Could you check a few things on this model? Use its own coordinates, in mm. Give positions to 0.01 mm unless a question says otherwise; leave off trailing zeros. Loops run counter-clockwise (first coordinate to the right, second up) from the corner with the lowest first, then second, coordinate; pieces in that order, holes last. Notation, with made-up numbers: (73, 45) -> (96, 45) arc R21 ccw to (96, 74) -> close; hole circle Ø7 at (70.25, -38.75). An arc over 180 degrees is marked (long way). Write item = value, one per line. Start each with the question number.
1) I want a section at D-D (x = -24). List the corners of the cut face in (y, z) for me.
2) I want a section at B-B (y = 25.5). List the corners of the cut face in (x, z) for me.
3) I'm going to push flat-ended pins straight in: pin 1 Ø18 at (x, y) = (0, 0) entering from +Z; pin 2 Ø3 at (y, z) = (28.5, 4.5) entering from -X. Where does each tip first touch, or does it pass through?
4) I want a section at A-A (x = 4). List the corners of the cut face in (y, z) for me.
5) I want a section at C-C (z = 5.5). List the corners of the cut face in (x, y) for me.
6) If we mould it in two halves opening along X, with no side actions, what happens to faces 1 (the face through (13.93, 40.2, 3.45)), 2 (the face through (-0.4, 11.4, 0)), 3 (the face through (-11.19, 0.49, 3.45))? For each: +X half, -X half, draft (parallel to the pull), parting line (faces both ways), or undercut.
7) I need wall thicknesses on probe 1 along Y at (x, z) = (-14, 5.75); probe 2 along Y at (x, z) = (0, 5.75); probe 3 along Y at (x, z) = (-2.5, 6). Which ranges of each line are inside material? Lowest first, please. Write a range as from..to.
from build123d import *

# Parameters (mm, degrees)
F0_R         = 11.2
F1_DEPTH     = 7
F2_T4_ANGLE  = 151.1667099625
F2_T10_ANGLE = 155.7575231718
F2_T16_ANGLE = 151.1667099625
F2_T22_ANGLE = 155.7575231718


# Not quite as in the source:
# - a fillet or chamfer that OpenCascade refuses, or shapes differently, is made with other operations: its cross-section is extruded or revolved along the edge and cut away or added


with BuildPart() as f1:
    # F0 (on Top) → F1 (new body)
    with BuildSketch(Plane.XY):
        with BuildLine():
            ThreePointArc((9.3591465956, -16.7270162039), (17.6571466732, 0.0595617509), (8.3139799998, 16.2876621091))
            Line((8.3139799998, 16.2876621091), (-9.3591465956, 16.7270162039))
            ThreePointArc((-9.3591465956, 16.7270162039), (-17.3223324531, -0.048962325), (-8.3139799998, -16.2876621091))
            Line((-8.3139799998, -16.2876621091), (9.3591465956, -16.7270162039))
        make_face()
        Circle(F0_R, mode=Mode.SUBTRACT)
        Polygon((8.3139799998, 16.2876621091), (27.5946892798, 32.5588136911), (-0.1261595724, 48.0615143736), (-27.5946892798, 33.4348380566), (-9.3591465956, 16.7270162039), align=None)
        with Locations((0, 31.6827967763)):
            Circle(F0_R, mode=Mode.SUBTRACT)
        Polygon((27.5946892798, -33.4348380566), (9.3591465956, -16.7270162039), (-8.3139799998, -16.2876621091), (-27.5946892798, -32.5588136911), (0.1261595724, -48.0615143736), align=None)
        with Locations((0, -31.6827967763)):
            Circle(F0_R, mode=Mode.SUBTRACT)
    extrude(amount=F1_DEPTH)

    # F2: fillet of radius 3 on 4 edges, made by hand


with BuildPart() as f2_tool2:
    # F2_s3 → F2_t4 (revolve)
    with BuildSketch(Plane(origin=(2.9031932082, 0.8450981198, 0), x_dir=(0, 0, 1), z_dir=(0.9601480198, 0.2794920035, 0))):
        with BuildLine():
            ThreePointArc((4, -20.0470026749), (6.1213203436, -19.1683230184), (7, -17.0470026749))
            Line((7, -17.0470026749), (7, -20.0470026749))
            Line((7, -20.0470026749), (4, -20.0470026749))
        make_face()
    revolve(axis=Axis((2.9763887281, 0.5936471566, 7), (0, 0, 1)), revolution_arc=F2_T4_ANGLE)

    split(bisect_by=Plane(origin=(4.0604237069, 4.4316985467, 0), x_dir=(0, 0, 1), z_dir=(-0.6755468125, -0.7373170987, 0)), keep=Keep.TOP)

    split(bisect_by=Plane(origin=(4.569745577, -5.414978498, 0), x_dir=(0, 0, 1), z_dir=(-0.6449416276, 0.7642318346, 0)), keep=Keep.TOP)


with BuildPart() as f1_1:
    add(f1.part)

    # F2_t1: cut F2_tool2
    add(f2_tool2.part, mode=Mode.SUBTRACT)


with BuildPart() as f2_tool8:
    # F2_s9 → F2_t10 (revolve)
    with BuildSketch(Plane(origin=(-2.2049800931, -0.547085883, 0), x_dir=(0, 0, 1), z_dir=(-0.9705717322, -0.2408121936, 0))):
        with BuildLine():
            ThreePointArc((4, -19.889257837), (6.1213203436, -19.0105781805), (7, -16.889257837))
            Line((7, -16.889257837), (7, -19.889257837))
            Line((7, -19.889257837), (4, -19.889257837))
        make_face()
    revolve(axis=Axis((-2.1995295918, -0.5690536346, 7), (0, 0, 1)), revolution_arc=F2_T10_ANGLE)

    split(bisect_by=Plane(origin=(-4.0604237069, -4.4316985467, 0), x_dir=(0, 0, 1), z_dir=(0.6755468125, 0.7373170987, 0)), keep=Keep.TOP)

    split(bisect_by=Plane(origin=(-4.569745577, 5.414978498, 0), x_dir=(0, 0, 1), z_dir=(0.6449416276, -0.7642318346, 0)), keep=Keep.TOP)


with BuildPart() as f1_2:
    add(f1_1.part)

    # F2_t7: cut F2_tool8
    add(f2_tool8.part, mode=Mode.SUBTRACT)


with BuildPart() as f2_tool14:
    # F2_s15 → F2_t16 (revolve)
    with BuildSketch(Plane(origin=(2.9031932082, 0.8450981198, 0), x_dir=(0, 0, 1), z_dir=(0.9601480198, 0.2794920035, 0))):
        with BuildLine():
            ThreePointArc((3, -20.0470026749), (0.8786796564, -19.1683230184), (0, -17.0470026749))
            Line((0, -17.0470026749), (0, -20.0470026749))
            Line((0, -20.0470026749), (3, -20.0470026749))
        make_face()
    revolve(axis=Axis((2.9763887281, 0.5936471566, 0), (0, 0, 1)), revolution_arc=F2_T16_ANGLE)

    split(bisect_by=Plane(origin=(4.0604237069, 4.4316985467, 0), x_dir=(0, 0, 1), z_dir=(-0.6755468125, -0.7373170987, 0)), keep=Keep.TOP)

    split(bisect_by=Plane(origin=(4.569745577, -5.414978498, 0), x_dir=(0, 0, 1), z_dir=(-0.6449416276, 0.7642318346, 0)), keep=Keep.TOP)


with BuildPart() as f1_3:
    add(f1_2.part)

    # F2_t13: cut F2_tool14
    add(f2_tool14.part, mode=Mode.SUBTRACT)


with BuildPart() as f2_tool20:
    # F2_s21 → F2_t22 (revolve)
    with BuildSketch(Plane(origin=(-2.2049800931, -0.547085883, 0), x_dir=(0, 0, 1), z_dir=(-0.9705717322, -0.2408121936, 0))):
        with BuildLine():
            ThreePointArc((3, -19.889257837), (0.8786796564, -19.0105781805), (0, -16.889257837))
            Line((0, -16.889257837), (0, -19.889257837))
            Line((0, -19.889257837), (3, -19.889257837))
        make_face()
    revolve(axis=Axis((-2.1995295918, -0.5690536346, 0), (0, 0, 1)), revolution_arc=F2_T22_ANGLE)

    split(bisect_by=Plane(origin=(-4.0604237069, -4.4316985467, 0), x_dir=(0, 0, 1), z_dir=(0.6755468125, 0.7373170987, 0)), keep=Keep.TOP)

    split(bisect_by=Plane(origin=(-4.569745577, 5.414978498, 0), x_dir=(0, 0, 1), z_dir=(0.6449416276, -0.7642318346, 0)), keep=Keep.TOP)


with BuildPart() as f1_4:
    add(f1_3.part)

    # F2_t19: cut F2_tool20
    add(f2_tool20.part, mode=Mode.SUBTRACT)


solid = f1_4.part
Answer list:
q1.outline = (-34.57, 0) -> (-29.53, 0) -> (-29.53, 7) -> (-34.57, 7) -> close; (30.14, 0) -> (35.35, 0) -> (35.35, 7) -> (30.14, 7) -> close
q2.outline = (-18.93, 0) -> (-9.34, 0) -> (-9.34, 7) -> (-18.93, 7) -> close; (9.34, 0) -> (19.23, 0) -> (19.23, 7) -> (9.34, 7) -> close
q3.pin_1 = through
q3.pin_2 = -23.85
q4.outline = (-46, 0) -> (-42.14, 0) -> (-42.14, 7) -> (-46, 7) -> close; (-21.22, 0) -> (-10.46, 0) -> (-10.46, 7) -> (-21.22, 7) -> close; (10.46, 0) -> (21.22, 0) -> (21.22, 7) -> (10.46, 7) -> close; (42.14, 0) -> (45.75, 0) -> (45.75, 7) -> (42.14, 7) -> close
q5.outline = (-27.59, -32.56) -> (0.13, -48.06) -> (27.59, -33.43) -> (9.06, -16.45) arc R19.46 ccw to (7.99, 16.01) -> (27.59, 32.56) -> (-0.13, 48.06) -> (-27.59, 33.43) -> (-9.06, 16.45) arc R19.91 ccw to (-7.99, -16.02) -> close; hole circle Ø22.4 at (0, -31.68); hole circle Ø22.4 at (0, 0); hole circle Ø22.4 at (0, 31.68)
q6.face_1 = +X half
q6.face_2 = draft
q6.face_3 = undercut
q7.probe_1 = -40.16..-21.09, -9.49..10.68, 20.98..40.67
q7.probe_2 = -47.99..-42.88, -20.48..-11.2, 11.2..20.48, 42.88..47.99
q7.probe_3 = -46.59..-42.6, -20.77..-10.92, 10.92..20.77, 42.6..46.8
